Here's how the part is built. I have some questions about the finished solid (model axes, mm). Face numbers are marked on the shaded views. A direction names the side the tool comes from. Coordinates: 2 decimals unless noted, no trailing zeros. Order: outer loops, then holes, each group sorted by start corner. A loop starts at its lowest first (then second) coordinate and runs counter-clockwise, first axis right, second up. Notation, with made-up numbers: (30, -30) - (79, -30) arc R26 cw to (79, -1) - close; hole circle Ø9 at (74.25, 29). An arc over 180 degrees is marked (long way). Answer in a Markdown table with one row per item. Add a question column.
Item 1: Will these pins go through, and if not, where does the flat tip stop? pin 1 Ø2.5 at (x, y) = (13, 34.5) entering from +Z; pin 2 Ø1.5 at (x, y) = (23, -22) entering from +Z; pin 3 Ø1 at (x, z) = (8, 6) entering from -Y.
Item 2: I want a section at B-B (y = 27.5). Please give me the cut outline in (x, z).
Item 3: I want a section at C-C (x = -34.5). Please give me the cut outline in (y, z).
Item 4: I want a section at D-D (y = -21.5). Please give me the cut outline in (x, z).
Item 5: On a 3-axis mill with a long thin cutter (end or side, diameter ignored), from which of +Z, -Z, +X, -X, +Y, -Y can I reach the whole of each face in a straight line? I mean the marked faces 1, 2 and 3. Say none if no direction works.
Item 6: Thinking about a two-plate mould opening in X: for the marked faces 4, 5 and 6, which applies, +X half, -X half, draft (parallel to the pull), parting line (faces both ways), or undercut?
Item 7: If I drill on line 1 along X through (y, z) = (26, 15); line 2 along Z through (x, y) = (-4, 10); line 3 along Y through (x, z) = (-62.5, 9.5), over which ranges is the centre line in solid material (lowest first)? Write a range as from..to.
```python
from build123d import *

# Parameters (mm, degrees)
F1_DEPTH     = 3
F0_W         = 2.7
F0_H         = 65
F2_DEPTH     = 16.4
F0_W_2       = 111
F0_H_2       = 3
F3_DEPTH     = 3.8
F4_W         = 24
F4_H         = 2.4
F5_DEPTH     = 1.5
F6_W         = 24
F6_H         = 2.4
F7_DEPTH     = 1.5
F8_T1_DEPTH  = 31.73221831
F8_T6_DEPTH  = 31.73221831
F8_T11_DEPTH = 31.73221831
F8_T16_DEPTH = 31.73221831
F9_F1_R      = 1.5
F9_F2_R      = 1.5
F9_F3_R      = 1.4999
F9_F4_R      = 1.4999
F9_F5_R      = 1.5
F9_F6_R      = 1.5
F9_F7_R      = 1.5
F9_F8_R      = 1.5
F9_F9_R      = 1.5
F9_F10_R     = 1.5
F9_F11_R     = 1.5
F9_F12_R     = 1.5


# Not quite as in the source:
# - a fillet or chamfer that OpenCascade refuses, or shapes differently, is made with other operations: its cross-section is extruded or revolved along the edge and cut away or added
# - a fillet or chamfer is up to 0.001 mm smaller than in the source, because OpenCascade refuses the exact size


with BuildPart() as f1:
    # F0 (on Top) → F1 (new body)
    with BuildSketch(Plane.XY):
        Polygon((-68.3, -32.5), (68.3, -32.5), (68.3, 32.5), (55.5, 32.5), (-55.5, 32.5), (-68.3, 32.5), align=None)
    extrude(amount=F1_DEPTH)

    # F0 (on Top) → F2 (join)
    with BuildSketch(Plane.XY):
        Polygon((-71, 32.5), (-68.3, 32.5), (-55.5, 32.5), (-55.5, 35.5), (-71, 35.5), align=None)
        with Locations((-69.65, 0)):
            Rectangle(F0_W, F0_H)
        Polygon((68.3, 32.5), (71, 32.5), (71, 35.5), (55.5, 35.5), (55.5, 32.5), align=None)
        with Locations((69.65, 0)):
            Rectangle(F0_W, F0_H)
    extrude(amount=F2_DEPTH)

    # F0 (on Top) → F3 (join)
    with BuildSketch(Plane.XY):
        with Locations((0, 34)):
            Rectangle(F0_W_2, F0_H_2)
    extrude(amount=F3_DEPTH)

    # F4 (on face) → F5 (join)
    with BuildSketch(Plane.YZ.offset(-68.3)):
        with Locations((-15, 9.2)):
            Rectangle(F4_W, F4_H)
    extrude(amount=F5_DEPTH)

    # F6 (on face) → F7 (join)
    with BuildSketch(Plane(origin=(68.3, 0, 0), x_dir=(0, -1, 0), z_dir=(-1, 0, 0))):
        with Locations((15, 9.2)):
            Rectangle(F6_W, F6_H)
    extrude(amount=F7_DEPTH)

    # F8: chamfer of 1.5 x 1.2586494468 on 4 edges, made by hand

    # F8_s2 → F8_t1 (cut)
    with BuildSketch(Plane.XZ.offset(-0.866109155)):
        Polygon((68.0586494468, 8), (66.8, 9.5), (66.8, 8), align=None)
    extrude(amount=F8_T1_DEPTH, mode=Mode.SUBTRACT)


with BuildPart() as f8_tool4:
    # F8_s5 → F8_t6 (new body)
    with BuildSketch(Plane.XZ.offset(-0.866109155)):
        Polygon((-68.3, 10.4), (-66.8, 9.1413505532), (-66.8, 10.4), align=None)
    extrude(amount=F8_T6_DEPTH)

    split(bisect_by=Plane.YZ.offset(-68.3), keep=Keep.TOP)


with BuildPart() as f1_1:
    add(f1.part)

    # F8_t3: cut F8_tool4
    add(f8_tool4.part, mode=Mode.SUBTRACT)


with BuildPart() as f8_tool9:
    # F8_s10 → F8_t11 (new body)
    with BuildSketch(Plane.XZ.offset(30.866109155)):
        Polygon((68.3, 10.4), (66.8, 9.1413505532), (66.8, 10.4), align=None)
    extrude(amount=-F8_T11_DEPTH)

    split(bisect_by=Plane.YZ.offset(68.3), keep=Keep.BOTTOM)


with BuildPart() as f1_2:
    add(f1_1.part)

    # F8_t8: cut F8_tool9
    add(f8_tool9.part, mode=Mode.SUBTRACT)


with BuildPart() as f8_tool14:
    # F8_s15 → F8_t16 (new body)
    with BuildSketch(Plane.XZ.offset(30.866109155)):
        Polygon((-68.3, 8), (-66.8, 9.2586494468), (-66.8, 8), align=None)
    extrude(amount=-F8_T16_DEPTH)

    split(bisect_by=Plane.YZ.offset(-68.3), keep=Keep.TOP)


with BuildPart() as f1_3:
    add(f1_2.part)

    # F8_t13: cut F8_tool14
    add(f8_tool14.part, mode=Mode.SUBTRACT)

    # F9: fillet of radius 1.5 on 12 edges, made by hand

    # F9_f1
    f9_f1_edges = [f1_3.edges().sort_by_distance(p)[0] for p in [
        (55.5, 35.5, 10.1),
    ]]
    fillet(f9_f1_edges, radius=F9_F1_R)

    # F9_f2
    f9_f2_edges = [f1_3.edges().sort_by_distance(p)[0] for p in [
        (-55.5, 35.5, 10.1),
    ]]
    fillet(f9_f2_edges, radius=F9_F2_R)

    # F9_f3 (radius 1.5 in the source; OpenCascade refuses exactly that, so slightly less here)
    f9_f3_edges = [f1_3.edges().sort_by_distance(p)[0] for p in [
        (-55.5, 32.5, 10.1),
    ]]
    fillet(f9_f3_edges, radius=F9_F3_R)

    # F9_f4 (radius 1.5 in the source; OpenCascade refuses exactly that, so slightly less here)
    f9_f4_edges = [f1_3.edges().sort_by_distance(p)[0] for p in [
        (55.5, 32.5, 10.1),
    ]]
    fillet(f9_f4_edges, radius=F9_F4_R)

    # F9_f5
    f9_f5_edges = [f1_3.edges().sort_by_distance(p)[0] for p in [
        (-68.3, -32.5, 9.7),
    ]]
    fillet(f9_f5_edges, radius=F9_F5_R)

    # F9_f6
    f9_f6_edges = [f1_3.edges().sort_by_distance(p)[0] for p in [
        (68.3, -32.5, 9.7),
    ]]
    fillet(f9_f6_edges, radius=F9_F6_R)

    # F9_f7
    f9_f7_edges = [f1_3.edges().sort_by_distance(p)[0] for p in [
        (-68.3, 32.5, 9.7),
    ]]
    fillet(f9_f7_edges, radius=F9_F7_R)

    # F9_f8
    f9_f8_edges = [f1_3.edges().sort_by_distance(p)[0] for p in [
        (68.3, 32.5, 9.7),
    ]]
    fillet(f9_f8_edges, radius=F9_F8_R)

    # F9_f9
    f9_f9_edges = [f1_3.edges().sort_by_distance(p)[0] for p in [
        (-71, -32.5, 8.2),
    ]]
    fillet(f9_f9_edges, radius=F9_F9_R)

    # F9_f10
    f9_f10_edges = [f1_3.edges().sort_by_distance(p)[0] for p in [
        (71, -32.5, 8.2),
    ]]
    fillet(f9_f10_edges, radius=F9_F10_R)

    # F9_f11
    f9_f11_edges = [f1_3.edges().sort_by_distance(p)[0] for p in [
        (-71, 35.5, 8.2),
    ]]
    fillet(f9_f11_edges, radius=F9_F11_R)

    # F9_f12
    f9_f12_edges = [f1_3.edges().sort_by_distance(p)[0] for p in [
        (71, 35.5, 8.2),
    ]]
    fillet(f9_f12_edges, radius=F9_F12_R)


solid = f1_3.part
```
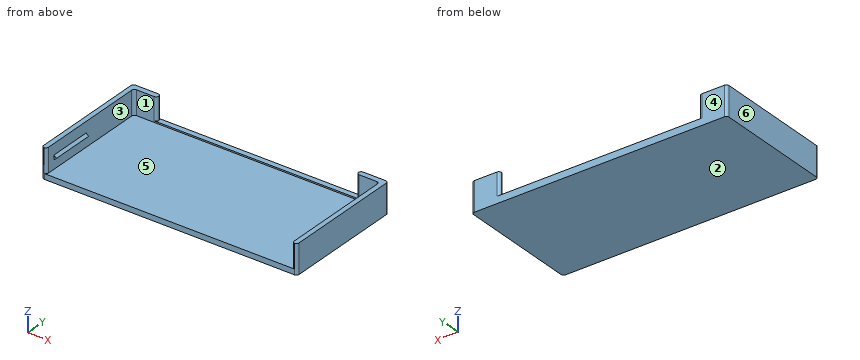
Values follow:
| question | item | result |
|---|---|---|
| 1 | pin 1 | stops at z = 3.8 |
| 1 | pin 2 | stops at z = 3 |
| 1 | pin 3 | passes through |
| 2 | outline | (-71, 0) - (71, 0) - (71, 16.4) - (68.3, 16.4) - (68.3, 3) - (-68.3, 3) - (-68.3, 16.4) - (-71, 16.4) - close |
| 3 | outline | (-32.5, 0) - (35.5, 0) - (35.5, 3.8) - (32.5, 3.8) - (32.5, 3) - (-32.5, 3) - close |
| 4 | outline | (-71, 0) - (71, 0) - (71, 16.4) - (68.3, 16.4) - (68.3, 10.4) - (66.98, 9.29) - (68.06, 8) - (68.3, 8) - (68.3, 3) - (-68.3, 3) - (-68.3, 8) - (-66.87, 9.2) - (-68.3, 10.4) - (-68.3, 16.4) - (-71, 16.4) - close |
| 5 | face 1 | +Z, -Y |
| 5 | face 2 | -Z, +X, -X, +Y, -Y |
| 5 | face 3 | none |
| 6 | face 4 | draft |
| 6 | face 5 | undercut |
| 6 | face 6 | -X half |
| 7 | line 1 | x = -71..-68.3, 68.3..71 |
| 7 | line 2 | z = 0..3 |
| 7 | line 3 | y = 32.5..35.5 |
